Could you check a few things on this model? Use its own coordinates, in mm. Coordinates: 2 decimals unless noted, no trailing zeros. Loops run counter-clockwise (first coordinate to the right, second up) from the corner with the lowest first, then second, coordinate; pieces in that order, holes last. Notation, with made-up numbers: M -28,54 L -2,54 A19 ccw -2,80 Z; hole C 34,-17 d2. An arc over 180 degrees is marked long. Write each question's results on one line, items separated by ' | '.
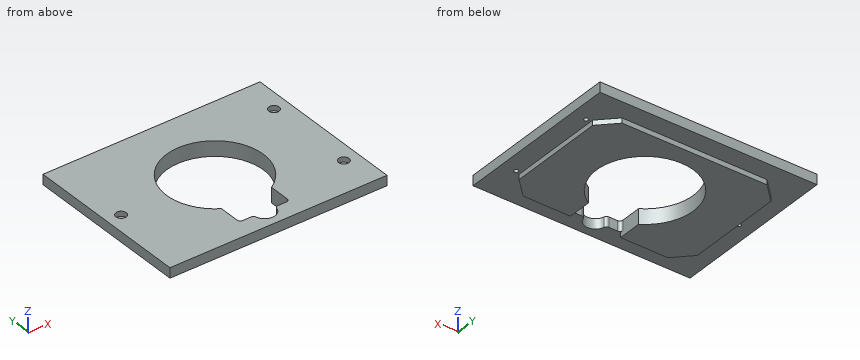
```python
from build123d import *

# Parameters (mm, degrees)
F0_W     = 260
F0_H     = 200
F1_DEPTH = 12
F2_DEPTH = 6
F3_R     = 6.15188
F3_R_2   = 2.4892
F4_DEPTH = 6
F5_DEPTH = 18.001
F6_R     = 3.81
F8_DEPTH = 18.001
F9_R     = 3.81


with BuildPart() as f1:
    # F0 (on Top) → F1 (new body)
    with BuildSketch(Plane.XY):
        Rectangle(F0_W, F0_H)
        Polygon((-86.75, 78), (86.75, 78), (106.75, 58), (106.75, -58), (86.75, -78), (30, -78), (-30, -78), (-86.75, -78), (-106.75, -58), (-106.75, 58), align=None, mode=Mode.SUBTRACT)
        with BuildLine():
            Line((106.75, 58), (86.75, 78))
            Line((86.75, 78), (-86.75, 78))
            Line((-86.75, 78), (-106.75, 58))
            Line((-106.75, 58), (-106.75, -58))
            Line((-106.75, -58), (-86.75, -78))
            Line((-86.75, -78), (-30, -78))
            Line((-30, -78), (-30, -49.638694584))
            ThreePointArc((-30, -49.638694584), (0, 58), (30, -49.638694584))
            Line((30, -49.638694584), (30, -78))
            Line((30, -78), (86.75, -78))
            Line((86.75, -78), (106.75, -58))
            Line((106.75, -58), (106.75, 58))
        make_face()
    extrude(amount=F1_DEPTH)

    # F0 (on Top) → F2 (join)
    with BuildSketch(Plane.XY):
        with BuildLine():
            Line((106.75, 58), (86.75, 78))
            Line((86.75, 78), (-86.75, 78))
            Line((-86.75, 78), (-106.75, 58))
            Line((-106.75, 58), (-106.75, -58))
            Line((-106.75, -58), (-86.75, -78))
            Line((-86.75, -78), (-30, -78))
            Line((-30, -78), (-30, -49.638694584))
            ThreePointArc((-30, -49.638694584), (0, 58), (30, -49.638694584))
            Line((30, -49.638694584), (30, -78))
            Line((30, -78), (86.75, -78))
            Line((86.75, -78), (106.75, -58))
            Line((106.75, -58), (106.75, 58))
        make_face()
    extrude(amount=-F2_DEPTH)

    # F3 (on face) → F4 (cut)
    with BuildSketch(Plane.XY.offset(12)):
        with Locations((-112.5, 0)):
            Circle(F3_R)
        with Locations((-112.5, 0)):
            Circle(F3_R_2, mode=Mode.SUBTRACT)
        with Locations((112.5, 55)):
            Circle(F3_R)
        with Locations((112.5, 55)):
            Circle(F3_R_2, mode=Mode.SUBTRACT)
        with Locations((112.5, -55)):
            Circle(F3_R)
        with Locations((112.5, -55)):
            Circle(F3_R_2, mode=Mode.SUBTRACT)
        with Locations((-112.5, 0)):
            Circle(F3_R_2)
        with Locations((112.5, 55)):
            Circle(F3_R_2)
        with Locations((112.5, -55)):
            Circle(F3_R_2)
    extrude(amount=-F4_DEPTH, mode=Mode.SUBTRACT)

    # F3 (on face) → F5 (cut, through all)
    with BuildSketch(Plane.XY.offset(12)):
        with Locations((-112.5, 0)):
            Circle(F3_R_2)
        with Locations((112.5, 55)):
            Circle(F3_R_2)
        with Locations((112.5, -55)):
            Circle(F3_R_2)
    extrude(amount=-F5_DEPTH, mode=Mode.SUBTRACT)

    # F6
    f6_edges = [f1.edges().sort_by_distance(p)[0] for p in [
        (-30, -78, 6),
        (30, -78, 6),
    ]]
    fillet(f6_edges, radius=F6_R)

    # F7 (on face) → F8 (cut, through all)
    with BuildSketch(Plane.XY.offset(12)):
        with BuildLine():
            Line((12.7, -78), (-12.7, -78))
            ThreePointArc((-12.7, -78), (0, -90.7), (12.7, -78))
        make_face()
    extrude(amount=-F8_DEPTH, mode=Mode.SUBTRACT)

    # F9
    f9_edges = [f1.edges().sort_by_distance(p)[0] for p in [
        (-12.7, -78, 6),
        (12.7, -78, 6),
    ]]
    fillet(f9_edges, radius=F9_R)


solid = f1.part
```
(1) Imagine slicing it at B-B, the plane y = -67. List the corners of the cut face in (x, z) for me, and give its area (3 significant figures).
Reported:
outline: M -130,0 L -97.75,0 L -97.75,-6 L -30,-6 L -30,12 L -130,12 Z; M 30,-6 L 97.75,-6 L 97.75,0 L 130,0 L 130,12 L 30,12 Z | area: 3,210 mm2
(2) Imagine slicing it at C-C, the plane z = 2.75. List the corners of the cut face in (x, y) for me, and give its area (3 significant figures).
Reported:
outline: M -130,-100 L 130,-100 L 130,100 L -130,100 Z; hole C -112.5,0 d4.98; hole M -30,-74.19 A3.81 ccw -26.19,-78 L -16.06,-78 A3.81 cw -12.36,-80.93 A12.7 ccw 12.36,-80.93 A3.81 cw 16.06,-78 L 26.19,-78 A3.81 ccw 30,-74.19 L 30,-49.64 A58 ccw long -30,-49.64 Z; hole C 112.5,-55 d4.98; hole C 112.5,55 d4.98 | area: 39,800 mm2
(3) Imagine slicing it at A-A, the plane x = 0. List the corners of the cut face in (y, z) for me.
Reported:
outline: M -100,0 L -90.7,0 L -90.7,12 L -100,12 Z; M 58,-6 L 78,-6 L 78,0 L 100,0 L 100,12 L 58,12 Z
(4) Will these pins go through, and if not, where does the flat tip stop? P1, Ø1.8, axis at x = 67.5, z = -4.5, coming from the -Y side; P2, Ø6, axis at x = 114, y = 56, coming from the +Z side; P3, Ø5, axis at y = 2.5, z = -4, coming from the +X side.
Reported:
P1: stops at y = -78 | P2: stops at z = 6 | P3: stops at x = 106.75
(5) Please list where these lines run through material, in increasing order: probe 1 along Y at (x, z) = (112.5, 9.8); probe 2 along Y at (x, z) = (112.5, 4.3); probe 3 along X at (y, z) = (-81, 8.5). Write a range as from..to.
Reported:
probe 1: y = -100..-61.15, -48.85..48.85, 61.15..100 | probe 2: y = -100..-57.49, -52.51..52.51, 57.49..100 | probe 3: x = -130..-12.34, 12.34..130
(6) Imagine slicing it at D-D, the plane y = 32.5. List the corners of the cut face in (x, z) for me.
Reported:
outline: M -130,0 L -106.75,0 L -106.75,-6 L -48.04,-6 L -48.04,12 L -130,12 Z; M 48.04,-6 L 106.75,-6 L 106.75,0 L 130,0 L 130,12 L 48.04,12 Z
